```python
from build123d import *

# Parameters (mm, degrees)
PRESS_KOVA_KAPAGI_KAPAK_1_START = 1340
PRESS_KOVA_KAPAGI_KAPAK_1_DEPTH = 440
PRESS_KOVA_KAPAGI_KAPAK_2_START = 27
SKETCH2_W                       = 26
SKETCH2_H                       = 180
PRESS_KOVA_KAPAGI_KAPAK_2_DEPTH = 14


with BuildPart() as part:
    # Sketch1 → PRESS_kova_kapagi_kapak_1 (new body)
    with BuildSketch(Plane(origin=(0, 0, 0), x_dir=(1, 0, 0), z_dir=(0, 1, 0)).offset(PRESS_KOVA_KAPAGI_KAPAK_1_START)):
        Polygon((30, -40), (30, -20), (31.5, -20), (31.5, -38.5), (338.5, -38.5), (338.5, -20), (340, -20), (340, -40), align=None)
    extrude(amount=PRESS_KOVA_KAPAGI_KAPAK_1_DEPTH)

    # Sketch2 → PRESS_kova_kapagi_kapak_2 (cut)
    with BuildSketch(Plane.XY.offset(PRESS_KOVA_KAPAGI_KAPAK_2_START)):
        with Locations((307, 1560)):
            Rectangle(SKETCH2_W, SKETCH2_H)
    extrude(amount=PRESS_KOVA_KAPAGI_KAPAK_2_DEPTH, mode=Mode.SUBTRACT)


solid = part.part
```
Verification items for the finished model (mm, model axes). A direction names the side the tool comes from. Give positions to 0.01 mm unless a question says otherwise; leave off trailing zeros. Order: outer loops, then holes, each group sorted by start corner. A loop starts at its lowest first (then second) coordinate and runs counter-clockwise, first axis right, second up. Notation, with made-up numbers: (74, -33.5) -> (124, -33.5) arc R21 ccw to (124, -12.5) -> close; hole circle Ø11 at (51.5, 87). An arc over 180 degrees is marked (long way). Use a Markdown table: item, result.
1) Depth check by flat-ended pin: pin 1 Ø10 at (x, y) = (276, 1513) entering from -Z. Enter the tip coordinate at first touch or a pass-through.
Results:
| item | result |
|---|---|
| pin 1 | z = 38.5 |
2) Section check C-C, the plane y = 1604. Record the boundary of the cut face in (x, z).
Results:
| item | result |
|---|---|
| outline | (30, 20) -> (31.5, 20) -> (31.5, 38.5) -> (294, 38.5) -> (294, 40) -> (30, 40) -> close; (320, 38.5) -> (338.5, 38.5) -> (338.5, 20) -> (340, 20) -> (340, 40) -> (320, 40) -> close |
3) Section check A-A, the plane x = 308. Record the boundary of the cut face in (y, z).
Results:
| item | result |
|---|---|
| outline | (1340, 38.5) -> (1470, 38.5) -> (1470, 40) -> (1340, 40) -> close; (1650, 38.5) -> (1780, 38.5) -> (1780, 40) -> (1650, 40) -> close |
4) Mould release check, pull along X, two halves, no side actions. Record for faces 1 (the flat face through (183, 1557, 38.5)), 2 (the flat face through (340, 1557, 30)), 3 (the flat face through (30, 1557, 30)): pulls with the +X half, pulls with the -X half, needs draft (parallel to the pull), parting line crosses it, or undercut.
Results:
| item | result |
|---|---|
| face 1 | undercut |
| face 2 | pulls with the +X half |
| face 3 | pulls with the -X half |
5) Material ranges on probe 1 along X at (y, z) = (1734, 28.5); probe 2 along Z at (x, y) = (77, 1660.5), recorded low to high.
Results:
| item | result |
|---|---|
| probe 1 | 30 to 31.5, 338.5 to 340 |
| probe 2 | 38.5 to 40 |
6) Tool access check on faces 4 (the flat face through (338.5, 1557, 29)), 5 (the flat face through (187, 1557, 40)). Record the directions out of +Z, -Z, +X, -X, +Y, -Y that give a thin tool (end or side, any length) a straight path to the whole face; none if there is none.
Results:
| item | result |
|---|---|
| face 4 | -Z, +Y, -Y |
| face 5 | +Z, +X, -X, +Y, -Y |
7) Section check B-B, the plane z = 28.25. Record the boundary of the cut face in (x, y).
Results:
| item | result |
|---|---|
| outline | (30, 1340) -> (31.5, 1340) -> (31.5, 1780) -> (30, 1780) -> close; (338.5, 1340) -> (340, 1340) -> (340, 1780) -> (338.5, 1780) -> close |
8) Section check D-D, the plane y = 1454. Record the boundary of the cut face in (x, z), then the cut area to 4 significant figures.
Results:
| item | result |
|---|---|
| outline | (30, 20) -> (31.5, 20) -> (31.5, 38.5) -> (338.5, 38.5) -> (338.5, 20) -> (340, 20) -> (340, 40) -> (30, 40) -> close |
| area | 520.5 mm² |
